from build123d import *

# Parameters (mm, degrees)
SKETCH1_R           = 5
BOSS_EXTRUDE1_DEPTH = 70
SKETCH2_R           = 2
CUT_EXTRUDE1_DEPTH  = 71
CUT_EXTRUDE2_DEPTH  = 3
LPATTERN1_COUNT     = 2
LPATTERN1_PITCH     = 67


with BuildPart() as part:
    # Sketch1 → Boss-Extrude1 (new body)
    with BuildSketch(Plane(origin=(0, 0, 0), x_dir=(1, 0, 0), z_dir=(0, 1, 0))):
        Circle(SKETCH1_R)
    extrude(amount=BOSS_EXTRUDE1_DEPTH)

    # Sketch2 → Cut-Extrude1 (cut, through all)
    with BuildSketch(Plane(origin=(0, 70, 0), x_dir=(1, 0, 0), z_dir=(0, 1, 0))):
        Circle(SKETCH2_R)
    extrude(amount=-CUT_EXTRUDE1_DEPTH, mode=Mode.SUBTRACT)

    # Sketch3 → Cut-Extrude2 (cut)
    with BuildSketch(Plane(origin=(0, 70, 0), x_dir=(1, 0, 0), z_dir=(0, 1, 0))):
        Polygon((1.599030575, -2.74343481), (3.175399526, 0.013083694), (1.576368951, 2.756518504), (-1.599030575, 2.74343481), (-3.175399526, -0.013083694), (-1.576368951, -2.756518504), align=None)
    cut_extrude2 = extrude(amount=-CUT_EXTRUDE2_DEPTH, mode=Mode.SUBTRACT)

    # LPattern1: Cut-Extrude2 ×2
    with Locations(*[(0, -i * LPATTERN1_PITCH, 0) for i in range(1, LPATTERN1_COUNT)]):
        add(cut_extrude2, mode=Mode.SUBTRACT)


solid = part.part
The model under review builds one solid part; all positions refer to its coordinate system, in mm. A direction names the side the tool comes from. Round coordinates to 2 decimals unless told otherwise and drop trailing zeros. Write each loop counter-clockwise with the first axis right and the second up, starting at its lowest first coordinate (ties: lowest second). Pieces come first, ordered by that corner, then holes. Notation, with made-up numbers: M 77.5,62.25 L 133.5,62.25 A26 ccw 133.5,83.25 Z; hole C 23,-11.75 d10. An arc over 180 degrees is marked long. Use a Markdown table: item, result. Add a question column.
Q1. We need section B-B, the plane z = 4. State the section outline as (x, y) points, plus the area to 3 significant figures.
Q2. Insertion check: pin 1 (1.5 mm diameter, centred on x = -2.5, y = 22, fed in from -Z); pin 2 (3 mm diameter, centred on x = 0.5, z = -0.5, fed in from +Y); pin 3 (3 mm diameter, centred on x = -3.5, z = -1, fed in from -Y); pin 4 (3.5 mm diameter, centred on x = 0, z = 0, fed in from +Y). Each pin has a flat end and moves straight along its axis. Give the tip position at first contact, or say it passes through.
Q3. The part is to be moulded in two halves that separate along Z. For faces 4 (the face through (-1.08, 34.51, 4.88)), 5 (the face through (2.2, 70, 2.2)), 6 (the face through (2.38, 68.52, 1.38)), say which applies: pulls with the +Z half, pulls with the -Z half, needs draft (parallel to the pull), parting line crosses it, or undercut.
Q4. Machinability: for faces 1 (the face through (2.2, 0, 2.2)), 2 (the face through (2, 3, -1)), 3 (the face through (-2.387, 68.521, 1.366)), which of the approach directions +Z, -Z, +X, -X, +Y, -Y give a long, thin tool a straight path to every point of the face, cutting with its end or side? Answer none if there is none.
Q5. We need section A-A, the plane x = 0.5. State the section outline as (y, z) points.
Q6. We need section C-C, the plane y = 38. State the section outline as (x, z) points.
Q7. We need section D-D, the plane x = 4. State the section outline as (y, z) points, plus the area to 3 significant figures.
Q8. To check wall thickness, follow line 1 (X direction, y = 25.5, z = 0); line 2 (Y direction, x = 1.25, z = -2). State the ranges of each line that lie inside material, in increasing order.
Findings below:
| question | item | result |
|---|---|---|
| 1 | outline | M -3,0 L 3,0 L 3,70 L -3,70 Z |
| 1 | area | 420 mm² |
| 2 | pin 1 | stops at z = -4.68 |
| 2 | pin 2 | stops at y = 67 |
| 2 | pin 3 | stops at y = 0 |
| 2 | pin 4 | passes through |
| 3 | face 4 | parting line crosses it |
| 3 | face 5 | needs draft |
| 3 | face 6 | undercut |
| 4 | face 1 | +Z, -Z, +X, -X, -Y |
| 4 | face 2 | -Y |
| 4 | face 3 | +Y |
| 5 | outline | M 0,-4.97 L 70,-4.97 L 70,-2.75 L 67,-2.75 L 67,-1.94 L 3,-1.94 L 3,-2.75 L 0,-2.75 Z; M 0,2.75 L 3,2.75 L 3,1.94 L 67,1.94 L 67,2.75 L 70,2.75 L 70,4.97 L 0,4.97 Z |
| 6 | outline | C 0,0 d10; hole C 0,0 d4 |
| 7 | outline | M 0,-3 L 70,-3 L 70,3 L 0,3 Z |
| 7 | area | 420 mm² |
| 8 | line 1 | x = -5 to -2, 2 to 5 |
| 8 | line 2 | y = 3 to 67 |
